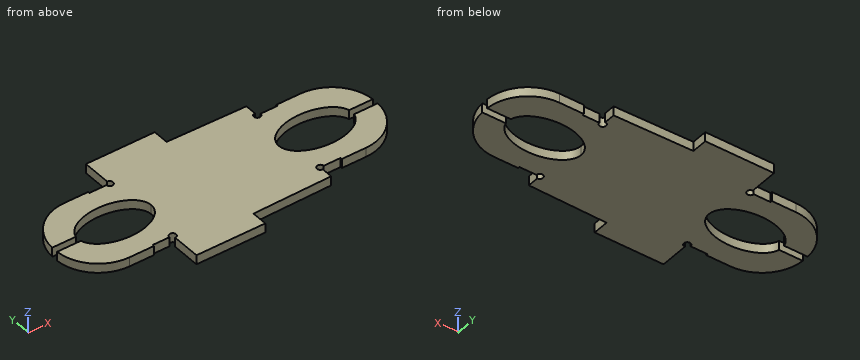
Autodesk Inventor part; units mm, degrees
ref_plane "YZ Plane" through (0, 0, 0) normal (1, 0, 0) x (0, 1, 0)
ref_plane "XZ Plane" through (0, 0, 0) normal (0, 1, 0) x (-1, 0, 0)
ref_plane "XY Plane" through (0, 0, 0) normal (0, 0, 1) x (1, 0, 0)
sketch "Sketch1" plane through (0, 0, 0) normal (0, 0, 1) x (1, 0, 0)
  line L0 (48.35, 0) -> (48.35, 13.2)
  line L1 (48.35, 13.2) -> (28.35, 13.2)
  line L2 (28.35, 13.2) -> (28.35, 12.7)
  line L3 (28.35, 12.7) -> (22.25, 12.7)
  line L4 (12.2521, 0) -> (48.35, 0)
  line L5 (22.25, 12.7) -> (22.25, 22.25)
  line L6 (22.25, 22.25) -> (0, 22.25)
  line L7 (48.35, 1) -> (41.2045, 1)
  line L8 (48.35, 0) -> (48.35, -13.2)
  line L9 (48.35, -13.2) -> (28.35, -13.2)
  line L10 (28.35, -13.2) -> (28.35, -12.7)
  line L11 (28.35, -12.7) -> (22.25, -12.7)
  line L12 (22.25, -12.7) -> (22.25, -22.25)
  line L13 (22.25, -22.25) -> (0, -22.25)
  line L14 (48.35, -1) -> (41.2045, -1)
  line L15 (0, 22.25) -> (0, -22.25)
  ellipse E0 centre (30.2836, 0) end of major axis (41.3256, 0) minor radius 6.7692 (41.2045, 1) -> (41.2045, -1) ccw
  point P0 (0, 0)
  point P1 (17.8114, 0)
  point P2 (41.275, 1)
  point P3 (41.275, -1)
  dimension "d0" = 13.2
  dimension "d1" = 20
  dimension "d6" = 12.7
  dimension "d7" = 22.25
  dimension "d8" = 22.25
  dimension "d9" = 6.1
  dimension "d17" = 48.35
  dimension "d34" = 1
extrude "Extrusion2" add sketch "Sketch1" along normal blind 2.794 contours L7 E0 L14 L8 L9 L10 L11 L12 L13 L15 L6 L5 L3 L2 L1 L0
pattern_circular "Circular Pattern1" count 2 over 360 about axis through (0, 0, -10) along (0, 0, 1) of "Extrusion2"
fillet "Fillet2" radius 12.7 2 edges at (48.35, 13.2, 1.397) (48.35, -13.2, 1.397)
fillet "Fillet3" radius 12.7 2 edges at (-48.35, -13.2, 1.397) (-48.35, 13.2, 1.397)
sketch "Sketch3" plane through (0, 0, 2.794) normal (0, 0, 1) x (1, 0, 0)
  line L0 (22.25, 12.7) -> (22.25, 22.25)
  line L1 (22.25, 22.25) -> (-22.25, 22.25)
  line L2 (-1.5, 17.5) -> (22.25, 17.0652)
  line L3 (22.25, 22.25) -> (22.25, 17.0652)
  line L4 (0, 0) -> (6.35, 0)
  line L5 (22.25, -12.7) -> (22.25, -22.25)
  line L6 (22.25, -22.25) -> (22.25, -17.0652)
  line L7 (-28.35, 13.2) -> (-35.6598, 13.2)
  line L8 (-1.5, 22.25) -> (-1.5, 17.5)
  line L9 (21.8285, 22.25) -> (-1.5, 22.25)
  line L10 (22.25, -12.7) -> (22.25, -22.25)
  line L11 (22.25, -22.25) -> (-22.25, -22.25)
  line L12 (-1.5, -17.5) -> (22.25, -17.0652)
  line L13 (-1.5, -22.25) -> (-1.5, -17.5)
  point P0 (0, 22.25)
  dimension "d32" = 1.5
  dimension "d33" = 17.5
extrude "Extrusion4" cut sketch "Sketch3" against normal up to next
hole "Hole1" at (22.2556, 12.6962, 2.794) direction (0, 0, -1) diameter 2 end through all
mirror "Mirror1" about plane through (0, 0, 0) normal (1, 0, 0) of "Hole1"
mirror "Mirror2" about plane through (0, 0, 0) normal (0, 1, 0) of "Hole1", "Mirror1"
equation "\"d7\" = d8"
properties part number "LockZ"
Read the model definition and answer for the solid it produces. Units are mm, in the model's axes. Round coordinates to 2 decimals unless told otherwise and drop trailing zeros. Write each loop counter-clockwise with the first axis right and the second up, starting at its lowest first coordinate (ties: lowest second). Pieces come first, ordered by that corner, then holes. Notation, with made-up numbers: (21.25, -17) - (55.25, -17) arc R25 ccw to (55.25, 12) - close; hole circle Ø2 at (28, 55.25). An arc over 180 degrees is marked (long way). Use a Markdown table: item, result.
(1) The part is cut by section B-B (x = 6.5). Write down the section's boundary in (y, z), then the cut area to 3 significant figures.
Reported:
| item | result |
|---|---|
| outline | (-17.35, 0) - (17.35, 0) - (17.35, 2.79) - (-17.35, 2.79) - close |
| area | 97.0 mm2 |
(2) Straight lines are drawn through the part: line 1 along X through (y, z) = (3.5, 2.4); line 2 along X through (y, z) = (-5.5, 0.2); line 3 along Y through (x, z) = (-30, 0.7). For each, find the intervals that lie inside material, in ascending order. Write a range as [from, to].
Reported:
| item | result |
|---|---|
| line 1 | [-47.99, -39.74], [-20.83, 20.83], [39.74, 47.99] |
| line 2 | [-47.32, -36.72], [-23.85, 23.85], [36.72, 47.32] |
| line 3 | [-13.2, -6.77], [6.77, 13.2] |
(3) The part is cut by section A-A (y = -3). State how many separate pieces and enclosed holes the cut face has, then the cut area to 3 significant figures.
Reported:
| item | result |
|---|---|
| separate pieces | 3 |
| enclosed holes | 0 |
| area | 158 mm2 |
(4) Each of these flat-tipped pins is pushed along its axis until it touches: pin 1 Ø0.8 at (x, z) = (45.5, 2) entering from +Y; pin 2 Ø1.4 at (x, z) = (32.5, 2) entering from +Y; pin 3 Ø1.6 at (x, y) = (-22.26, 12.7) entering from -Z; pin 4 Ø0.8 at (y, z) = (15.5, 2) entering from +X. Where does it stop, or does it pass through?
Reported:
| item | result |
|---|---|
| pin 1 | y = 8.98 |
| pin 2 | y = 13.2 |
| pin 3 | through |
| pin 4 | x = 22.25 |
